from build123d import *

# Parameters (mm, degrees)
SKIZZE1_R                            = 10
AUFSATZ_LINEAR_AUSTRAGEN1_DEPTH      = 2
SKIZZE4_R                            = 1
SCHNITT_LINEAR_AUSTRAGEN1_DEPTH      = 2
KREISMUSTER1_COUNT                   = 4
SKIZZE5_R                            = 4.5
AUFSATZ_LINEAR_AUSTRAGEN2_DEPTH      = 10
SKIZZE6_R                            = 8
AUFSATZ_LINEAR_AUSTRAGEN3_DEPTH      = 1
SKIZZE7_R                            = 1
SCHNITT_LINEAR_AUSTRAGEN2_DEPTH      = 5
SCHNITT_LINEAR_AUSTRAGEN2_DEPTH_BACK = 5


with BuildPart() as part:
    # Skizze1 → Aufsatz-Linear austragen1 (new body)
    with BuildSketch(Plane.XY):
        Circle(SKIZZE1_R)
    extrude(amount=AUFSATZ_LINEAR_AUSTRAGEN1_DEPTH)

    # Skizze4 → Schnitt-Linear austragen1 (cut)
    with BuildSketch(Plane.XY.offset(2)):
        with Locations((-8, 0)):
            Circle(SKIZZE4_R)
    schnitt_linear_austragen1 = extrude(amount=-SCHNITT_LINEAR_AUSTRAGEN1_DEPTH, mode=Mode.SUBTRACT)

    # Kreismuster1: Schnitt-Linear austragen1 ×4 about axis
    kreismuster1_axis = Axis((0.080808081, 0, 0), (0, 0, 1))
    for i in range(1, KREISMUSTER1_COUNT):
        add(schnitt_linear_austragen1.rotate(kreismuster1_axis, i * 360 / KREISMUSTER1_COUNT), mode=Mode.SUBTRACT)

    # Skizze5 → Aufsatz-Linear austragen2 (add)
    with BuildSketch(Plane.XY.offset(2)):
        Circle(SKIZZE5_R)
    extrude(amount=AUFSATZ_LINEAR_AUSTRAGEN2_DEPTH)

    # Skizze6 → Aufsatz-Linear austragen3 (add)
    with BuildSketch(Plane.XY.offset(12)):
        Circle(SKIZZE6_R)
    extrude(amount=AUFSATZ_LINEAR_AUSTRAGEN3_DEPTH)

    # Skizze7 → Schnitt-Linear austragen2 (cut, two sides)
    with BuildSketch(Plane(origin=(0, 0, 0), x_dir=(0, 0, -1), z_dir=(1, 0, 0))) as schnitt_linear_austragen2_sk:
        with Locations((-9.972447251, 0)):
            Circle(SKIZZE7_R)
        with Locations((-6.278379976, 0)):
            Circle(SKIZZE7_R)
    extrude(amount=SCHNITT_LINEAR_AUSTRAGEN2_DEPTH, mode=Mode.SUBTRACT)
    extrude(schnitt_linear_austragen2_sk.sketch, amount=-SCHNITT_LINEAR_AUSTRAGEN2_DEPTH_BACK, mode=Mode.SUBTRACT)


solid = part.part
Read the model definition and answer for the solid it produces. Units are mm, in the model's axes. A direction names the side the tool comes from. Round coordinates to 2 decimals unless told otherwise and drop trailing zeros. Write each loop counter-clockwise with the first axis right and the second up, starting at its lowest first coordinate (ties: lowest second). Pieces come first, ordered by that corner, then holes.
Q1. A tool of negligible diameter and unlimited length cuts with its end or side. For faces 5 (the face through (-2.17, -9.76, 0.99)), 6 (the face through (4.292, 1.352, 6.93)), 7 (the face through (0, 0, 0)), 8 (the face through (7.208, -0.3, 1.014)), 9 (the face through (-1.73, -7.81, 12.49)), from which of +Z, -Z, +X, -X, +Y, -Y can it reach the whole face along a straight path? Write none if from no direction.
Values:
face 5: +Z, -Z
face 6: none
face 7: -Z, +X, -X, +Y, -Y
face 8: -Z
face 9: +Z
Q2. Find section D-D on y = -6.75. Determine the outline of the cut face in (x, z).
Values:
outline: (-7.38, 0) - (7.38, 0) - (7.38, 2) - (-7.38, 2) - close; (-4.29, 12) - (4.29, 12) - (4.29, 13) - (-4.29, 13) - close
Q3. Find section A-A on y = 0. Determine the outline of the cut face in (x, z).
Values:
outline: (-10, 0) - (-9, 0) - (-9, 2) - (-10, 2) - close; (-8, 12) - (-4.5, 12) - (-4.5, 10.97) - (4.5, 10.97) - (4.5, 12) - (8, 12) - (8, 13) - (-8, 13) - close; (-7, 0) - (7.16, 0) - (7.16, 2) - (4.5, 2) - (4.5, 5.28) - (-4.5, 5.28) - (-4.5, 2) - (-7, 2) - close; (-4.5, 7.28) - (4.5, 7.28) - (4.5, 8.97) - (-4.5, 8.97) - close; (9.16, 0) - (10, 0) - (10, 2) - (9.16, 2) - close
Q4. The mould has two halves that part along Z. Classify faces 1 (the face through (0.12, 9.08, 1.01)), 2 (the face through (0, 0, 13)), 3 (the face through (3.4, -3.4, 12)), 4 (the face through (-5, 0, 2)): released by +Z, released by -Z, zero draft, split by the parting line, or undercut.
Values:
face 1: zero draft
face 2: released by +Z
face 3: undercut
face 4: undercut
Q5. Find section B-B on x = -0.5. Determine the outline of the cut face in (y, z).
Values:
outline: (-9.99, 0) - (-8.89, 0) - (-8.89, 2) - (-9.99, 2) - close; (-7.98, 12) - (-4.47, 12) - (-4.47, 2) - (-7.27, 2) - (-7.27, 0) - (7.27, 0) - (7.27, 2) - (4.47, 2) - (4.47, 12) - (7.98, 12) - (7.98, 13) - (-7.98, 13) - close; (8.89, 0) - (9.99, 0) - (9.99, 2) - (8.89, 2) - close; hole circle Ø2 at (0, 6.28); hole circle Ø2 at (0, 9.97)
Q6. Flat-ended cylindrical pins translate along their axes: P1, Ø2, axis at y = -7, z = 5, coming from the -X side; P2, Ø1.5, axis at x = 3, z = 4, coming from the +Y side; P3, Ø6, axis at x = -6.5, z = 1.5, coming from the +Y side. Find the tip coordinate at first contact, or state that the pin passes through.
Values:
P1: passes through
P2: stops at y = 3.9
P3: stops at y = 9.37
Q7. Straight lines are drawn through the part: line 1 (Z direction, x = -3, y = 6); line 2 (Z direction, x = 3.75, y = -0.25); line 3 (Z direction, x = -6, y = 5.5). For each, find the intervals that lie inside material, in ascending order.
Values:
line 1: z = 0 to 2, 12 to 13
line 2: z = 0 to 5.31, 7.25 to 9, 10.94 to 13
line 3: z = 0 to 2
Q8. Find section C-C on x = 5. Determine the outline of the cut face in (y, z) (3 decimals), and give its area (3 significant figures).
Values:
outline: (-8.66, 0) - (8.66, 0) - (8.66, 2) - (-8.66, 2) - close; (-6.245, 12) - (6.245, 12) - (6.245, 13) - (-6.245, 13) - close
area: 47.1 mm2
